The model under review builds one solid part; all positions refer to its coordinate system, in mm. A direction names the side the tool comes from. Coordinates: 2 decimals unless noted, no trailing zeros. Order: outer loops, then holes, each group sorted by start corner. A loop starts at its lowest first (then second) coordinate and runs counter-clockwise, first axis right, second up. Notation, with made-up numbers: M 43.25,52.5 L 91.25,52.5 A20 cw 91.25,59.5 Z; hole C 87,51 d1. An arc over 180 degrees is marked long. One line per item, written item: value.
Autodesk Inventor part; units mm, degrees
ref_plane "YZ Plane" through (0, 0, 0) normal (1, 0, 0) x (0, 1, 0)
ref_plane "XZ Plane" through (0, 0, 0) normal (0, 1, 0) x (-1, 0, 0)
ref_plane "XY Plane" through (0, 0, 0) normal (0, 0, 1) x (1, 0, 0)
sketch "Sketch1" plane through (0, 0, 0) normal (0, 0, 1) x (1, 0, 0)
  circle A0 centre (0, 0) radius 49.2125
  circle A1 centre (0, 0) radius 6.35
  circle A2 centre (0, 0) radius 36.5125
  circle A3 centre (0, 0) radius 12.7
  line L0 (-1.5875, 7.9375) -> (1.5875, 7.9375)
  line L1 (1.5875, 7.9375) -> (1.5875, 6.1484)
  line L2 (1.5875, 6.1484) -> (-1.5875, 6.1484)
  line L3 (-1.5875, 6.1484) -> (-1.5875, 7.9375)
  point P0 (0, 6.1484)
  dimension "d1" = 12.7
  dimension "d0" = 98.425
  dimension "d2" = 12.7
  dimension "d3" = 25.4
  dimension "d10" = 7.9375
  dimension "d11" = 3.175
extrude "Extrusion1" add sketch "Sketch1" along normal mid plane 20.32 contours A0
extrude "Extrusion2" add sketch "Sketch1" along normal mid plane 15.24 contours A2
extrude "Extrusion3" add sketch "Sketch1" along normal mid plane 20.32 contours L2 A1 | A1 L3 L0 L1 | A3 picked at (-0.1781, 6.2081)
extrude "Extrusion4" cut sketch "Sketch1" along normal mid plane 25.4 contours L2 A1 | A1 L3 L0 L1 picked at (-0.1781, 6.2081)
properties part number "wheel"
(1) We need section D-D, the plane y = 16.5. State the section outline as (x, z) points.
Geometry results:
outline: M -46.36,-10.16 L -32.57,-10.16 L -32.57,-7.62 L 32.57,-7.62 L 32.57,-10.16 L 46.36,-10.16 L 46.36,10.16 L 32.57,10.16 L 32.57,7.62 L -32.57,7.62 L -32.57,10.16 L -46.36,10.16 Z
(2) We need section B-B, the plane x = 0. State the section outline as (y, z) points.
Geometry results:
outline: M -49.21,-10.16 L -36.51,-10.16 L -36.51,-7.62 L -12.7,-7.62 L -12.7,-10.16 L -6.35,-10.16 L -6.35,10.16 L -12.7,10.16 L -12.7,7.62 L -36.51,7.62 L -36.51,10.16 L -49.21,10.16 Z; M 7.94,-10.16 L 12.7,-10.16 L 12.7,-7.62 L 36.51,-7.62 L 36.51,-10.16 L 49.21,-10.16 L 49.21,10.16 L 36.51,10.16 L 36.51,7.62 L 12.7,7.62 L 12.7,10.16 L 7.94,10.16 Z
(3) Insertion check: pin 1 Ø5 at (x, z) = (36.5, -3) entering from +Y; pin 2 Ø1 at (x, y) = (21.5, 3) entering from +Z; pin 3 Ø0.9 at (y, z) = (7.5, 4) entering from -X. Each pin has a flat end and moves straight along its axis. Give the tip position at first contact, or say it passes through.
Geometry results:
pin 1: stops at y = 35.58
pin 2: stops at z = 7.62
pin 3: stops at x = -48.7
(4) We need section A-A, the plane y = 0. State the section outline as (x, z) points.
Geometry results:
outline: M -49.21,-10.16 L -36.51,-10.16 L -36.51,-7.62 L -12.7,-7.62 L -12.7,-10.16 L -6.35,-10.16 L -6.35,10.16 L -12.7,10.16 L -12.7,7.62 L -36.51,7.62 L -36.51,10.16 L -49.21,10.16 Z; M 6.35,-10.16 L 12.7,-10.16 L 12.7,-7.62 L 36.51,-7.62 L 36.51,-10.16 L 49.21,-10.16 L 49.21,10.16 L 36.51,10.16 L 36.51,7.62 L 12.7,7.62 L 12.7,10.16 L 6.35,10.16 Z
(5) For L1, parallel to Y at x = 0, z = -9.1; L2, parallel to Y at x = 0, z = -5.25; L3, parallel to Y at x = 5, z = -9.25, list the stretches that pass through material, from the lowest coordinate up.
Geometry results:
L1: y = -49.21 to -36.51, -12.7 to -6.35, 7.94 to 12.7, 36.51 to 49.21
L2: y = -49.21 to -6.35, 7.94 to 49.21
L3: y = -48.96 to -36.17, -11.67 to -3.91, 3.91 to 11.67, 36.17 to 48.96
(6) We need section C-C, the plane x = -32. State the section outline as (y, z) points, plus the area to 3 significant figures.
Geometry results:
outline: M -37.39,-10.16 L -17.58,-10.16 L -17.58,-7.62 L 17.58,-7.62 L 17.58,-10.16 L 37.39,-10.16 L 37.39,10.16 L 17.58,10.16 L 17.58,7.62 L -17.58,7.62 L -17.58,10.16 L -37.39,10.16 Z
area: 1,340 mm2
(7) Mouldability with a two-part tool opening along Y and no side actions: class faces 5 (the flat face through (3, 6, -10.16)), 6 (the cylindrical face through (46.94, -14.78, -0.14)), 7 (the flat face through (-1, -16, -7.62)), 8 (the cylindrical face through (0.257, -6.345, -0.142)) as +Y half, -Y half, draft (parallel to the pull), parting line (faces both ways), or undercut.
Geometry results:
face 5: draft
face 6: parting line
face 7: undercut
face 8: undercut
(8) Tool access review of faces 1 (the cylindrical face through (-2.75, -12.4, -8.87)), 2 (the cylindrical face through (34.826, -10.967, 8.872)), 3 (the flat face through (0, 7.938, 0)), 4 (the flat face through (0, 37, -10.16)): name each direction out of +Z, -Z, +X, -X, +Y, -Y from which nothing blocks a thin tool from reaching the whole face with its end or side.
Geometry results:
face 1: -Z
face 2: +Z
face 3: +Z, -Z
face 4: -Z, +X, -X, +Y, -Y
